Part model, mm, in its own coordinate system. Face numbers are marked on the shaded views. A direction names the side the tool comes from. Give positions to 0.01 mm unless a question says otherwise; leave off trailing zeros. Write each loop counter-clockwise with the first axis right and the second up, starting at its lowest first coordinate (ties: lowest second). Pieces come first, ordered by that corner, then holes. Notation, with made-up numbers: M 13.25,-18 L 22.25,-18 A21 ccw 22.25,1 Z; hole C -30,34 d10. An arc over 180 degrees is marked long. Answer as CSV lines item,"result". Start each with the question number.
1) Slice it at D-D, the plane z = 13. Give the cut face in (x, y) (3 decimals), plus the area to 3 significant figures.
2) Pin check, flat tips, straight feed: pin 1 Ø6.5 at (x, y) = (34.925, 0) entering from +Z (1 decimal); pin 2 Ø15 at (x, y) = (0, 34.925) entering from +Z. Stop position of each tip, or through.
3) Tool access for the marked faces 1 and 2: list every direction of +Z, -Z, +X, -X, +Y, -Y with a clear straight run to the whole face (end or side of a thin tool).
4) Slice it at B-B, the plane x = 0. Give the cut face in (y, z) (3 decimals).
5) Slice it at C-C, the plane z = 4.5. Give the cut face in (x, y) (3 decimals), plus the area to 3 significant figures.
6) Mould opens along X. For the marked faces 3, 4, 5 and 6 say: pulls with the +X half, pulls with the -X half, needs draft (parallel to the pull), parting line crosses it, or undercut.
7) Wall check: line 1 along Y through (x, z) = (0, 14) (3 decimals); line 2 along Y through (x, z) = (0, 4); line 3 along X through (y, z) = (3, 13). Give the ranges that are in metal, low to high. Write a range as from..to.
8) Slice it at A-A, the plane y = 0. Give the cut face in (x, z) (3 decimals).
```python
from build123d import *

# Parameters (mm, degrees)
F0_W           = 152.4
F0_H           = 152.4
F1_DEPTH       = 19.05
F3_D           = 8.4328
F4_D           = 10.3124
F4_CBORE_D     = 19.05
F4_CBORE_DEPTH = 12.7
F5_SIZE        = 6.35


with BuildPart() as f1:
    # F0 (on Top) → F1 (new body)
    with BuildSketch(Plane.XY):
        Rectangle(F0_W, F0_H)
    extrude(amount=F1_DEPTH)

    # F3 (through all)
    with Locations(Plane.XY.offset(19.05)):
        with Locations((-34.925, 0), (34.925, 0)):
            Hole(F3_D / 2)

    # F4 (through all)
    with Locations(Plane.XY.offset(19.05)):
        with Locations((0, 34.925), (0, 0), (0, -34.925)):
            CounterBoreHole(F4_D / 2, F4_CBORE_D / 2, F4_CBORE_DEPTH)

    # F5
    f5_edges = [f1.edges().sort_by_distance(p)[0] for p in [
        (-76.2, 76.2, 9.525),
        (-76.2, -76.2, 9.525),
        (76.2, -76.2, 9.525),
        (76.2, 76.2, 9.525),
    ]]
    chamfer(f5_edges, length=F5_SIZE)


solid = f1.part
```
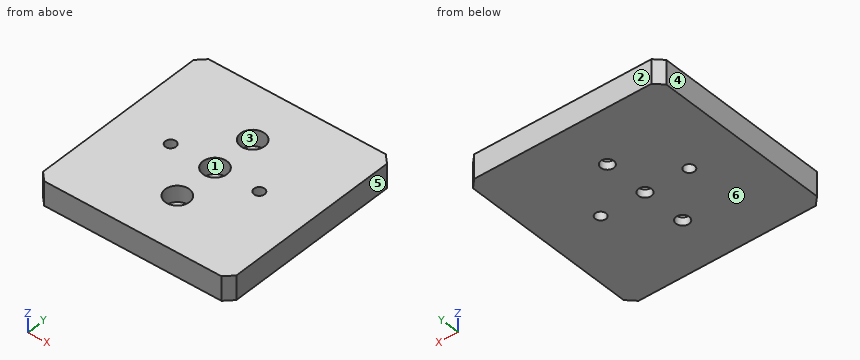
Found:
1,outline,"M -76.2,-69.85 L -69.85,-76.2 L 69.85,-76.2 L 76.2,-69.85 L 76.2,69.85 L 69.85,76.2 L -69.85,76.2 L -76.2,69.85 Z; hole C -34.925,0 d8.433; hole C 0,-34.925 d19.05; hole C 0,0 d19.05; hole C 0,34.925 d19.05; hole C 34.925,0 d8.433"
1,area,"22,200 mm²"
2,pin 1,"through"
2,pin 2,"z = 6.35"
3,face 1,"+Z"
3,face 2,"+Z, -Z, +X, -X, +Y"
4,outline,"M -76.2,0 L -40.081,0 L -40.081,6.35 L -44.45,6.35 L -44.45,19.05 L -76.2,19.05 Z; M -29.769,0 L -5.156,0 L -5.156,6.35 L -9.525,6.35 L -9.525,19.05 L -25.4,19.05 L -25.4,6.35 L -29.769,6.35 Z; M 5.156,0 L 29.769,0 L 29.769,6.35 L 25.4,6.35 L 25.4,19.05 L 9.525,19.05 L 9.525,6.35 L 5.156,6.35 Z; M 40.081,0 L 76.2,0 L 76.2,19.05 L 44.45,19.05 L 44.45,6.35 L 40.081,6.35 Z"
5,outline,"M -76.2,-69.85 L -69.85,-76.2 L 69.85,-76.2 L 76.2,-69.85 L 76.2,69.85 L 69.85,76.2 L -69.85,76.2 L -76.2,69.85 Z; hole C -34.925,0 d8.433; hole C 0,-34.925 d10.312; hole C 0,0 d10.312; hole C 0,34.925 d10.312; hole C 34.925,0 d8.433"
5,area,"22,800 mm²"
6,face 3,"undercut"
6,face 4,"pulls with the -X half"
6,face 5,"pulls with the +X half"
6,face 6,"needs draft"
7,line 1,"-76.2..-44.45, -25.4..-9.525, 9.525..25.4, 44.45..76.2"
7,line 2,"-76.2..-40.08, -29.77..-5.16, 5.16..29.77, 40.08..76.2"
7,line 3,"-76.2..-37.89, -31.96..-9.04, 9.04..31.96, 37.89..76.2"
8,outline,"M -76.2,0 L -39.141,0 L -39.141,19.05 L -76.2,19.05 Z; M -30.709,0 L -5.156,0 L -5.156,6.35 L -9.525,6.35 L -9.525,19.05 L -30.709,19.05 Z; M 5.156,0 L 30.709,0 L 30.709,19.05 L 9.525,19.05 L 9.525,6.35 L 5.156,6.35 Z; M 39.141,0 L 76.2,0 L 76.2,19.05 L 39.141,19.05 Z"
